Design review of the part built by this model. Coordinates are the model's own, in mm. A direction names the side the tool comes from. Round coordinates to 2 decimals unless told otherwise and drop trailing zeros. Loops run counter-clockwise (first coordinate to the right, second up) from the corner with the lowest first, then second, coordinate; pieces in that order, holes last. Notation, with made-up numbers: (-38.75, -10.5) - (-1.75, -10.5) arc R24 cw to (-1.75, 4.5) - close; hole circle Ø6 at (-26, 26). An arc over 180 degrees is marked (long way). Use one line per item in the form item = value. Start each with the question number.
(1) We need section B-B, the plane y = 0. Write out the cut boundary in (x, z), then the cut area to 4 significant figures.
(2) We need section C-C, the plane z = 7.25. Write out the cut boundary in (x, y).
(3) For pin 1 (4.5 mm diameter, centred on x = -7.05, y = 9.71, fed in from -Z); pin 2 (3.5 mm diameter, centred on x = 9.4, y = -12.94, fed in from +Z) (1 decimal); pin 3 (1.2 mm diameter, centred on x = -6.5, y = 10.5, fed in from +Z); pin 4 (8 mm diameter, centred on x = -2.5, z = 11.5, fed in from -Y), all flat-tipped, find the tip position at first contact; note any pin that passes through.
(4) We need section A-A, the plane x = 0. Write out the cut boundary in (y, z), then the cut area to 3 significant figures.
(5) Machinability: for faces 4 (the cylindrical face through (0, -14, 9)), 5 (the cylindrical face through (0.1, 12.5, 9.9)), 6 (the flat face through (-7, 7, 14)), 7 (the cylindrical face through (13.56, 3.42, 2.96)), 8 (the cylindrical face through (-9, 12, 10)), which of the approach directions +Z, -Z, +X, -X, +Y, -Y give a long, thin tool a straight path to every point of the face, cutting with its end or side? Answer none if there is none.
(6) We need section D-D, the plane y = -12. Write out the cut boundary in (x, z).
(7) The part is to be moulded in two halves that separate along Y. For faces 1 (the cylindrical face through (-0.1, -17.5, 5.8)), 2 (the cylindrical face through (-11.87, 3.92, 9.94)), 3 (the cylindrical face through (-16.683, -5.285, 5.754)), say which applies: released by +Y, released by -Y, zero draft, split by the parting line, or undercut.
(8) Wall thickness on probe 1 along Y at (x, z) = (0, 4.45); probe 2 along Y at (x, z) = (0, 3); probe 3 along Y at (x, z) = (-7, 10): over which ranges is each line inside the solid? List them lowest first. Write a range as [from, to].
Autodesk Fusion 360 part; units mm, degrees
sketch "Sketch1" plane through (0, 0, 0) normal (0, 0, 1) x (1, 0, 0)
  circle A0 centre (0, 0) radius 9
  circle A1 centre (0, 0) radius 16 construction
  line L0 (0, 0) -> (0, 16) construction
  circle A2 centre (0, 16) radius 3.5
  circle A3 centre (-15.2169, 4.9443) radius 3.5
  circle A4 centre (-9.4046, -12.9443) radius 3.5
  circle A5 centre (9.4046, -12.9443) radius 3.5
  circle A6 centre (15.2169, 4.9443) radius 3.5
  circle A7 centre (0, 0) radius 15
  circle A8 centre (0, 0) radius 21
  circle A9 centre (0, 0) radius 12 construction
  line L1 (0, 0) -> (-8.8168, 12.1353) construction
  circle A10 centre (-7.0534, 9.7082) radius 2
  circle A11 centre (-7.0534, 9.7082) radius 2.25 construction
  circle A12 centre (-11.4127, -3.7082) radius 2
  circle A13 centre (0, -12) radius 2
  circle A14 centre (11.4127, -3.7082) radius 2
  circle A15 centre (7.0534, 9.7082) radius 2
  line L2 (0, 0) -> (-15.2169, 4.9443) construction
  circle A16 centre (0, 16) radius 2.25
  circle A17 centre (-15.2169, 4.9443) radius 2.25
  circle A18 centre (-9.4046, -12.9443) radius 2.25
  circle A19 centre (9.4046, -12.9443) radius 2.25
  circle A20 centre (15.2169, 4.9443) radius 2.25
  circle A21 centre (0, 0) radius 8.5
  dimension "d1" = 18
  dimension "d3" = 7
  dimension "d5" = 360
  dimension "d6" = 30
  dimension "d7" = 42
  dimension "d8" = 4
  dimension "d9" = 4.5
  dimension "d10" = 24
  dimension "d12" = 360
  dimension "d13" = 36
  dimension "d14" = 72
  dimension "d17" = 4.5
  dimension "d19" = 360
  dimension "d26" = 17
  dimension "d31" = 32
extrude "Extrude1" add sketch "Sketch1" along normal blind 6 contours A2 A3 A4 A5 A6 A7 | A8
extrude "Extrude6" add sketch "Sketch1" along normal blind 14 contours A2 A3 A4 A5 A6 A7
extrude "Extrude7" add sketch "Sketch1" along normal blind 6 contours A2 A7 A16 | A2 A7 A16 | A3 A7 A17 | A3 A7 A17 | A6 A7 A20 | A6 A7 A20 | A4 A7 A18 | A4 A7 A18 | A5 A7 A19 | A5 A7 A19
extrude "Extrude4" add sketch "Sketch1" along normal blind 14 contours A0
extrude "Extrude5" cut sketch "Sketch1" along normal blind 4 contours A0
sketch "Sketch2" plane through (0, 0, 6) normal (0, 0, 1) x (-1, 0, 0)
  circle A0 centre (0, 0) radius 21
  arc A1 (-12.9338, -7.5971) -> (-3.2285, -14.6484) centre (0, 0) ccw
  arc A2 (-12.9338, -7.5971) -> (-14.9292, -1.4561) centre (-15.2169, -4.9443) ccw
  arc A3 (-11.2221, 9.9532) -> (-14.9292, -1.4561) centre (0, 0) ccw
  arc A4 (-11.2221, 9.9532) -> (-5.9982, 13.7485) centre (-9.4046, 12.9443) ccw
  arc A5 (5.9982, 13.7485) -> (-5.9982, 13.7485) centre (0, 0) ccw
  arc A6 (5.9982, 13.7485) -> (11.2221, 9.9532) centre (9.4046, 12.9443) ccw
  arc A7 (14.9292, -1.4561) -> (11.2221, 9.9532) centre (0, 0) ccw
  arc A8 (14.9292, -1.4561) -> (12.9338, -7.5971) centre (15.2169, -4.9443) ccw
  arc A9 (3.2285, -14.6484) -> (12.9338, -7.5971) centre (0, 0) ccw
  arc A10 (3.2285, -14.6484) -> (-3.2285, -14.6484) centre (0, -16) ccw
  circle A11 centre (0, 0) radius 17.5
  circle A12 centre (9.4046, 12.9443) radius 2.25
  circle A13 centre (15.2169, -4.9443) radius 2.25
  circle A14 centre (-9.4046, 12.9443) radius 2.25
  circle A15 centre (0, -16) radius 2.25
  circle A16 centre (-15.2169, -4.9443) radius 2.25
  dimension "d36" = 35
extrude "Extrude8" cut sketch "Sketch2" against normal blind 0.5 contours A0
sketch "Sketch3" plane through (0, 0, 0) normal (0, 0, -1) x (1, 0, 0)
  circle A0 centre (0, 0) radius 9
  circle A1 centre (-9.4046, 12.9443) radius 2.25
  circle A2 centre (-15.2169, -4.9443) radius 2.25
  circle A3 centre (9.4046, 12.9443) radius 2.25
  circle A4 centre (0, -16) radius 2.25
  circle A5 centre (15.2169, -4.9443) radius 2.25
  circle A6 centre (-7.0534, -9.7082) radius 2
  circle A7 centre (11.4127, 3.7082) radius 2
  circle A8 centre (0, 12) radius 2
  circle A9 centre (7.0534, -9.7082) radius 2
  circle A10 centre (-11.4127, 3.7082) radius 2
  circle A11 centre (0, 0) radius 21
extrude "Extrude9" add sketch "Sketch3" against normal blind 4 contours A6 | A7 | A8 | A9 | A10
equation "d10 = ( d6 - d1 ) / 2 + d1"
equation "d13 = d14 / 2"
Data:
q1.outline = (-21, 0) - (-9, 0) - (-9, 4) - (-8.5, 4) - (-8.5, 14) - (-15, 14) - (-15, 6) - (-17.5, 6) - (-17.5, 5.5) - (-21, 5.5) - close; (8.5, 4) - (9, 4) - (9, 0) - (21, 0) - (21, 5.5) - (17.5, 5.5) - (17.5, 6) - (15, 6) - (15, 14) - (8.5, 14) - close
q1.area = 246.5 mm^2
q2.outline = (-14.93, 1.46) arc R15 ccw to (-11.22, -9.95) arc R3.5 cw to (-6, -13.75) arc R15 ccw to (6, -13.75) arc R3.5 cw to (11.22, -9.95) arc R15 ccw to (14.93, 1.46) arc R3.5 cw to (12.93, 7.6) arc R15 ccw to (3.23, 14.65) arc R3.5 cw to (-3.23, 14.65) arc R15 ccw to (-12.93, 7.6) arc R3.5 cw to start; hole circle Ø4 at (-11.41, -3.71); hole circle Ø4 at (-7.05, 9.71); hole circle Ø17 at (0, 0); hole circle Ø4 at (0, -12); hole circle Ø4 at (7.05, 9.71); hole circle Ø4 at (11.41, -3.71)
q3.pin_1 = 0
q3.pin_2 = through
q3.pin_3 = 4
q3.pin_4 = -15
q4.outline = (-21, 0) - (-9, 0) - (-9, 4) - (-8.5, 4) - (-8.5, 14) - (-10, 14) - (-10, 4) - (-14, 4) - (-14, 14) - (-15, 14) - (-15, 6) - (-17.5, 6) - (-17.5, 5.5) - (-21, 5.5) - close; (8.5, 4) - (9, 4) - (9, 0) - (13.75, 0) - (13.75, 6) - (12.5, 6) - (12.5, 14) - (8.5, 14) - close; (18.25, 0) - (21, 0) - (21, 5.5) - (18.25, 5.5) - close
q4.area = 160 mm^2
q5.face_4 = +Z
q5.face_5 = +Z, +Y
q5.face_6 = +Z, +X, -X, +Y, -Y
q5.face_7 = +Z, -Z
q5.face_8 = +Z, -X, +Y
q6.outline = (-17.23, 0) - (-11.45, 0) - (-11.45, 6) - (-12.74, 6) - (-12.74, 5.5) - (-17.23, 5.5) - close; (-7.36, 0) - (7.36, 0) - (7.36, 6) - (6.03, 6) - (6.03, 14) - (2, 14) - (2, 4) - (-2, 4) - (-2, 14) - (-6.03, 14) - (-6.03, 6) - (-7.36, 6) - close; (11.45, 0) - (17.23, 0) - (17.23, 5.5) - (12.74, 5.5) - (12.74, 6) - (11.45, 6) - close
q7.face_1 = released by -Y
q7.face_2 = undercut
q7.face_3 = split by the parting line
q8.probe_1 = [-21, -14], [-10, -8.5], [8.5, 13.75], [18.25, 21]
q8.probe_2 = [-21, -9], [9, 13.75], [18.25, 21]
q8.probe_3 = [-10.4, -4.82], [4.82, 7.71], [11.71, 13.27]
